from build123d import *

# Parameters (mm, degrees)
BOSS_EXTRUDE1_DEPTH     = 5
BOSS_EXTRUDE2_DEPTH     = 13
CUT_EXTRUDE1_START      = -13
SKETCH3_R               = 2.3
CUT_EXTRUDE1_DEPTH      = 7.5
SKETCH4_R               = 1.65
BOSS_EXTRUDE3_DEPTH     = 6
CUT_EXTRUDE2_DEPTH      = 86.071137152
CUT_EXTRUDE2_DEPTH_BACK = 10
SKETCH9_R               = 1.65
CUT_EXTRUDE3_DEPTH      = 6


with BuildPart() as part:
    # Sketch1 → Boss-Extrude1 (new body)
    with BuildSketch(Plane(origin=(0, 0, 0), x_dir=(0, 0, -1), z_dir=(1, 0, 0))):
        with BuildLine():
            Line((-34.593659354, 3.256520294), (-46.7897518, -6.296129983))
            ThreePointArc((-46.7897518, -6.296129983), (-33.290290023, -15.004245976), (-18.234604608, -20.60719958))
            Line((-18.234604608, -20.60719958), (-2.973495544, 21.32235297))
            Line((-2.973495544, 21.32235297), (-17.068884855, 26.45265512))
            Line((-17.068884855, 26.45265512), (-27.166620772, -1.290646299))
            ThreePointArc((-27.166620772, -1.290646299), (-30.963724442, 0.846415848), (-34.593659354, 3.256520294))
        make_face()
    extrude(amount=BOSS_EXTRUDE1_DEPTH)

    # Sketch2 → Boss-Extrude2 (add)
    with BuildSketch(Plane(origin=(5, 0, 0), x_dir=(0, 0, -1), z_dir=(1, 0, 0))):
        with BuildLine():
            Line((-34.593659354, 3.256520294), (-46.7897518, -6.296129983))
            ThreePointArc((-46.7897518, -6.296129983), (-42.613802597, -9.444548196), (-38.226724688, -12.291412509))
            Line((-38.226724688, -12.291412509), (-25.335917908, -2.194623762))
            ThreePointArc((-25.335917908, -2.194623762), (-26.255160174, -1.750514609), (-27.166620772, -1.290646299))
            ThreePointArc((-27.166620772, -1.290646299), (-30.963724442, 0.846415848), (-34.593659354, 3.256520294))
        make_face()
        with BuildLine():
            Line((-25.335917908, -2.194623762), (-38.226724688, -12.291412509))
            ThreePointArc((-38.226724688, -12.291412509), (-28.535215176, -17.181480963), (-18.234604608, -20.60719958))
            Line((-18.234604608, -20.60719958), (-12.16072752, -3.919359432))
            Line((-12.16072752, -3.919359432), (-2.973495544, 21.32235297))
            Line((-2.973495544, 21.32235297), (-17.068884855, 26.45265512))
            Line((-17.068884855, 26.45265512), (-26.256116832, 1.210942718))
            Line((-26.256116832, 1.210942718), (-27.166620772, -1.290646299))
            ThreePointArc((-27.166620772, -1.290646299), (-26.255160174, -1.750514609), (-25.335917908, -2.194623762))
        make_face()
    extrude(amount=BOSS_EXTRUDE2_DEPTH)

    # Sketch3 → Cut-Extrude1 (cut)
    with BuildSketch(Plane(origin=(18, 0, 0), x_dir=(0, 0, -1), z_dir=(1, 0, 0)).offset(CUT_EXTRUDE1_START)):
        with Locations((-40.691705577, -1.519804845)):
            Circle(SKETCH3_R)
    extrude(amount=CUT_EXTRUDE1_DEPTH, mode=Mode.SUBTRACT)

    # Sketch4 → Boss-Extrude3 (add)
    with BuildSketch(Plane(origin=(18, 0, 0), x_dir=(0, 0, -1), z_dir=(1, 0, 0))):
        with BuildLine():
            Line((-13.371212035, 36.611927698), (-21.083585591, 15.422355502))
            ThreePointArc((-21.083585591, 15.422355502), (-19.723042607, 9.989582455), (-14.174598147, 9.227437939))
            ThreePointArc((-14.174598147, 9.227437939), (-10.385594526, 10.792784565), (-6.423166383, 11.844460235))
            Line((-6.423166383, 11.844460235), (1.530859032, 33.697965455))
            Line((1.530859032, 33.697965455), (9.165031814, 33.697965455))
            ThreePointArc((9.165031814, 33.697965455), (9.933965272, 34.117264651), (10.683756157, 34.569905907))
            Line((10.683756157, 34.569905907), (13.30556247, 36.552911383))
            ThreePointArc((13.30556247, 36.552911383), (13.786023096, 36.997313573), (14.25164947, 37.457235089))
            Line((14.25164947, 37.457235089), (14.25164947, 45.3641606))
            Line((14.25164947, 45.3641606), (24.03628358, 48.30778647))
            ThreePointArc((24.03628358, 48.30778647), (26.349985315, 51.429769983), (24.017555191, 54.53778647))
            Line((24.017555191, 54.53778647), (14.241296463, 57.414910041))
            ThreePointArc((14.241296463, 57.414910041), (0, 66.87164947), (-14.241296463, 57.414910041))
            Line((-14.241296463, 57.414910041), (-24.017555191, 54.53778647))
            ThreePointArc((-24.017555191, 54.53778647), (-26.349985315, 51.429769983), (-24.03628358, 48.30778647))
            Line((-24.03628358, 48.30778647), (-14.25164947, 45.3641606))
            Line((-14.25164947, 45.3641606), (-14.25164947, 37.457235089))
            ThreePointArc((-14.25164947, 37.457235089), (-13.817896207, 37.027847242), (-13.371212035, 36.611927698))
        make_face()
        with BuildLine():
            Line((7.5, 51.42), (7.981152097, 51.42))
            Line((7.981152097, 51.42), (7.064819397, 48.902396598))
            ThreePointArc((7.064819397, 48.902396598), (-7.390404098, 52.697469085), (7.5, 51.42))
        make_face(mode=Mode.SUBTRACT)
        with Locations((16.22, 51.42)):
            Circle(SKETCH4_R, mode=Mode.SUBTRACT)
        with Locations((-16.22, 51.42)):
            Circle(SKETCH4_R, mode=Mode.SUBTRACT)
    extrude(amount=BOSS_EXTRUDE3_DEPTH)

    # Sketch8 → Cut-Extrude2 (cut, two sides: drawn at the far end of the back side and taken through both)
    with BuildSketch(Plane.ZY.offset(-CUT_EXTRUDE2_DEPTH_BACK)):
        Polygon((17.068884855, -17.404410883), (17.068884855, 16.982887384), (8.814387371, 23.448263736), (2.973495544, 21.32235297), align=None)
        Polygon((8.814387371, 23.448263736), (17.068884855, 16.982887384), (17.068884855, 26.45265512), align=None)
        Polygon((17.068884855, 16.982887384), (21.890012849, 13.206714822), (17.068884855, 26.45265512), align=None)
    extrude(amount=CUT_EXTRUDE2_DEPTH + CUT_EXTRUDE2_DEPTH_BACK, mode=Mode.SUBTRACT)

    # Sketch9 → Cut-Extrude3 (cut)
    with BuildSketch(Plane.ZY):
        with Locations((24.568884855, -6.047927384)):
            Circle(SKETCH9_R)
        with Locations((37.335347169, -3.97184687)):
            Circle(SKETCH9_R)
        with Locations((21.576904852, -15.17107203)):
            Circle(SKETCH9_R)
    extrude(amount=-CUT_EXTRUDE3_DEPTH, mode=Mode.SUBTRACT)


solid = part.part
Design review of the part built by this model. Coordinates are the model's own, in mm. A direction names the side the tool comes from. Round coordinates to 2 decimals unless told otherwise and drop trailing zeros. Write each loop counter-clockwise with the first axis right and the second up, starting at its lowest first coordinate (ties: lowest second). Pieces come first, ordered by that corner, then holes.
Item 1: Consider section B-B on x = 20.75. Give the boundary of the cut face in (y, z), and give its area (3 significant figures).
Item 2: Consider section C-C on z = 41. Give the boundary of the cut face in (x, y), and give its area (3 significant figures).
Item 3: Wall thickness on L1, parallel to Y at x = 21.4, z = -16.22; L2, parallel to X at y = 54, z = 20; L3, parallel to X at y = 3, z = 10.5: over which ranges is each line inside the solid? List them lowest first.
Item 4: Draft analysis for pull direction Y (two halves, no side actions). For faces 1 (the cylindrical face through (20.96, 49.81, 16.58)), 2 (the flat face through (0, -6, 29)), 3 (the flat face through (8.87, -3.58, 43.32)), state which applies: released by +Y, released by -Y, zero draft, split by the parting line, or undercut.
Item 5: For faces 4 (the flat face through (21, 41, -14.252)), 5 (the flat face through (20.96, 50.18, -7.53)), 6 (the cylindrical face through (20.958, 10.774, 10.44)), 7 (the flat face through (6, -6, 25)), list the 3-axis set-ups (+Z, -Z, +X, -X, +Y, -Y) from which the entire face can be reached by the end or side of a thin tool; tool diameter is ignored.
Item 6: Consider section D-D on z = 0. Give the boundary of the cut face in (x, y), and give its area (3 significant figures).
Item 7: Consider section A-A on z = -16.22. Give the boundary of the cut face in (x, y).
Item 8: For pin 1 Ø1.8 at (x, z) = (20, -6) entering from -Y; pin 2 Ø4.5 at (y, z) = (51.42, -16.22) entering from -X; pin 3 Ø11 at (y, z) = (-3, 28) entering from +X; pin 4 Ø2.5 at (y, z) = (51.42, 16.22) entering from -X, all flat-tipped, find the tip position at first contact; note any pin that passes through.
Check values:
1. outline: (9.23, 14.17) arc R31 cw to (11.84, 6.42) - (33.7, -1.53) - (33.7, -9.17) arc R19.95 ccw to (34.57, -10.68) - (36.55, -13.31) arc R19.95 ccw to (37.46, -14.25) - (45.36, -14.25) - (48.31, -24.04) arc R3.25 ccw to (54.54, -24.02) - (57.41, -14.24) arc R15.45 ccw to (57.41, 14.24) - (54.54, 24.02) arc R3.25 ccw to (48.31, 24.04) - (45.36, 14.25) - (37.46, 14.25) arc R19.95 ccw to (36.61, 13.37) - (15.42, 21.08) arc R5 ccw to start; hole (48.9, -7.06) - (51.42, -7.98) - (51.42, -7.5) arc R7.5 ccw (long way) to start; hole circle Ø3.3 at (51.42, -16.22); hole circle Ø3.3 at (51.42, 16.22)
1. area: 1,240 mm2
2. outline: (0, -10.54) - (18, -10.54) - (18, -1.76) - (12.5, -1.76) - (12.5, -3.8) - (5, -3.8) - (5, -1.76) - (0, -1.76) - close
2. area: 143 mm2
3. L1: y = 45.96 to 49.77, 53.07 to 56.83
3. L2: x = 18 to 24
3. L3: x = 10 to 18
4. face 1: undercut
4. face 2: zero draft
4. face 3: released by +Y
5. face 4: -Z, +X, -X, -Y
5. face 5: +X, -X
5. face 6: -Z, +X, -Y
5. face 7: -X
6. outline: (18, 29.49) - (24, 29.49) - (24, 43.92) - (18, 43.92) - close; (18, 58.92) - (24, 58.92) - (24, 66.87) - (18, 66.87) - close
6. area: 134 mm2
7. outline: (18, 45.96) - (24, 45.96) - (24, 49.77) - (18, 49.77) - close; (18, 53.07) - (24, 53.07) - (24, 56.83) - (18, 56.83) - close
8. pin 1: stops at y = 33.7
8. pin 2: stops at x = 18
8. pin 3: stops at x = 18
8. pin 4: passes through
